Model file for the job. Use its own axes, mm. Coordinates: 2 decimals unless noted, no trailing zeros. Write each loop counter-clockwise with the first axis right and the second up, starting at its lowest first coordinate (ties: lowest second). Pieces come first, ordered by that corner, then holes. Notation, with made-up numbers: M -39.5,-37.75 L 3.5,-37.75 A21 ccw 3.5,-12.75 Z; hole C 35,-28.75 d10. An arc over 180 degrees is marked long. Answer in a Markdown table with one row per item. Add a question column.
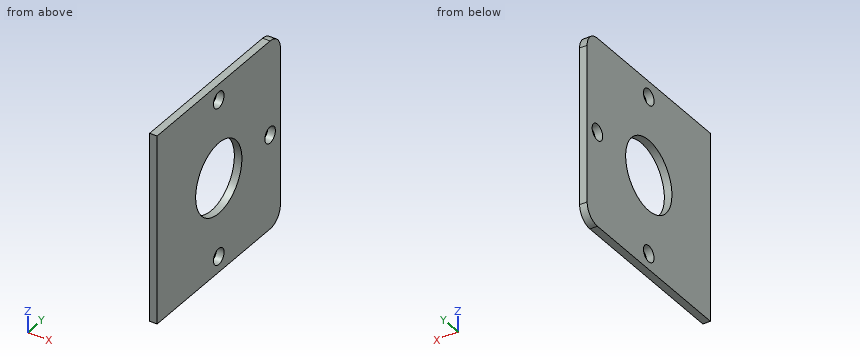
```python
from build123d import *

# Parameters (mm, degrees)
SKETCH1_W                 = 38.1
SKETCH1_H                 = 38.1
SKETCH1_R                 = 7.1501
BOSS_EXTRUDE1_DEPTH       = 1.524
F_4_CLEARANCE_HOLE1_D     = 3.2639
F_4_CLEARANCE_HOLE1_DEPTH = 1.524
FILLET1_R                 = 3.175


with BuildPart() as part:
    # Sketch1 → Boss-Extrude1 (new body)
    with BuildSketch(Plane(origin=(0, 0, 0), x_dir=(0, 0, -1), z_dir=(1, 0, 0))):
        Rectangle(SKETCH1_W, SKETCH1_H)
        Circle(SKETCH1_R, mode=Mode.SUBTRACT)
    extrude(amount=BOSS_EXTRUDE1_DEPTH)

    # #4 Clearance Hole1
    with Locations(Plane(origin=(1.524, 0, 0), x_dir=(0, 0, -1), z_dir=(1, 0, 0))):
        with Locations((-15.875, 0), (15.875, 0), (0, 15.875)):
            Hole(F_4_CLEARANCE_HOLE1_D / 2, depth=F_4_CLEARANCE_HOLE1_DEPTH)

    # Fillet1
    fillet1_edges = [part.edges().sort_by_distance(p)[0] for p in [
        (0.762, 19.05, 19.05),
        (0.762, 19.05, -19.05),
    ]]
    fillet(fillet1_edges, radius=FILLET1_R)


solid = part.part
```
1) Slice it at C-C (y = -5.5). Give the cut face in (x, z), then the cut area to 3 significant figures.
2) Drill centre lines: probe 1 along Y at (x, z) = (1.15, 0); probe 2 along Y at (x, z) = (0.5, -1); probe 3 along Y at (x, z) = (0.9, 17). Where is each one in solid material? Low to high.
3) Slice it at A-A (y = 0). Give the cut face in (x, z), then the cut area to 3 significant figures.
4) Slice it at B-B (z = 0). Give the cut face in (x, y).
5) Slice it at D-D (x = 1). Give the cut face in (y, z) (3 decimals).
6) Flat gauge pin, fed straight in: pin 1 Ø2 at (y, z) = (15.875, 0) entering from +X. Where does the tip first touch, or does it go through?
Ans:
| question | item | result |
|---|---|---|
| 1 | outline | M 0,-19.05 L 1.52,-19.05 L 1.52,-4.57 L 0,-4.57 Z; M 0,4.57 L 1.52,4.57 L 1.52,19.05 L 0,19.05 Z |
| 1 | area | 44.1 mm2 |
| 2 | probe 1 | y = -19.05 to -7.15, 7.15 to 14.24, 17.51 to 19.05 |
| 2 | probe 2 | y = -19.05 to -7.08, 7.08 to 14.59, 17.16 to 19.05 |
| 2 | probe 3 | y = -19.05 to -1.18, 1.18 to 18.84 |
| 3 | outline | M 0,-19.05 L 1.52,-19.05 L 1.52,-17.51 L 0,-17.51 Z; M 0,-14.24 L 1.52,-14.24 L 1.52,-7.15 L 0,-7.15 Z; M 0,7.15 L 1.52,7.15 L 1.52,14.24 L 0,14.24 Z; M 0,17.51 L 1.52,17.51 L 1.52,19.05 L 0,19.05 Z |
| 3 | area | 26.3 mm2 |
| 4 | outline | M 0,-19.05 L 1.52,-19.05 L 1.52,-7.15 L 0,-7.15 Z; M 0,7.15 L 1.52,7.15 L 1.52,14.24 L 0,14.24 Z; M 0,17.51 L 1.52,17.51 L 1.52,19.05 L 0,19.05 Z |
| 5 | outline | M -19.05,-19.05 L 15.875,-19.05 A3.175 ccw 19.05,-15.875 L 19.05,15.875 A3.175 ccw 15.875,19.05 L -19.05,19.05 Z; hole C 0,0 d14.3; hole C 0,-15.875 d3.264; hole C 0,15.875 d3.264; hole C 15.875,0 d3.264 |
| 6 | pin 1 | passes through |
